Model file for the job. Use its own axes, mm. A direction names the side the tool comes from. Give positions to 0.01 mm unless a question says otherwise; leave off trailing zeros. Order: outer loops, then holes, each group sorted by start corner. A loop starts at its lowest first (then second) coordinate and runs counter-clockwise, first axis right, second up. Notation, with made-up numbers: M 34.5,78.5 L 60.5,78.5 A33 cw 60.5,113.5 Z; hole C 59,73 d4. An arc over 180 degrees is marked long. Return JSON: item names as keys, results as strings. Group by question number.
1. 3-axis set-ups, long thin cutter, end or side, ignore diameter. For faces 1 (the face through (-1, 0, 70)), 2 (the face through (-99, -4, 75)), 3 (the face through (-50, -25, 71)), 4 (the face through (98, -4, 105)): which of +Z, -Z, +X, -X, +Y, -Y reach the whole face in a straight line?
2. Wall check: probe 1 along X at (y, z) = (-3, 104); probe 2 along X at (y, z) = (1, -89); probe 3 along X at (y, z) = (4.5, 29.74). Give the ranges that are in metal, low to high. Write a range as [from, to].
3. Slice it at B-B on z = 70. List the corners of the cut face in (x, y), then the cut area to 3 significant figures.
4. Slice it at C-C on y = -21.5. List the corners of the cut face in (x, z), then the cut area to 3 significant figures.
5. Slice it at D-D on x = -102. List the corners of the cut face in (y, z).
6. Two-plate mould, pull along X, no slides. Class faces 5 (the face through (-71.45, -4, 90)), 6 (the face through (-99, -4, 105)), 7 (the face through (-125, 2, 27)), 8 (the face through (40.25, -12, 24)): released by +X, released by -X, zero draft, split by the parting line, or undercut.
7. Pin check, flat tips, straight feed: pin 1 (12 mm diameter, centred on x = -29, z = 37.5, fed in from -Y); pin 2 (12.5 mm diameter, centred on x = -4, y = -8.5, fed in from -Z); pin 3 (2 mm diameter, centred on x = 111, y = -2, fed in from +Z). Stop position of each tip, or through.
8. Slice it at A-A on x = 0. List the corners of the cut face in (y, z).
from build123d import *

# Parameters (mm, degrees)
SKETCH1_W           = 250
SKETCH1_H           = 250
BOSS_EXTRUDE1_DEPTH = 8
SKETCH2_W           = 53.55
SKETCH2_H           = 30
BOSS_EXTRUDE2_DEPTH = 7.5
SKETCH3_R           = 2.25
CUT_EXTRUDE1_DEPTH  = 178.454923854
SKETCH4_R           = 1.5
BOSS_EXTRUDE3_DEPTH = 25
FILLET1_R           = 3
CUT_EXTRUDE2_REACH  = 219.518
SKETCH5_W           = 20
SKETCH5_H           = 10
SKETCH6_R           = 1.85096309
SKETCH6_R_2         = 7.5
CUT_EXTRUDE3_DEPTH  = 20
FILLET2_R           = 10


with BuildPart() as part:
    # Sketch1 → Boss-Extrude1 (new body)
    with BuildSketch(Plane(origin=(0, 0, 0), x_dir=(1, 0, 0), z_dir=(0, 1, 0))):
        Rectangle(SKETCH1_W, SKETCH1_H)
    extrude(amount=BOSS_EXTRUDE1_DEPTH)

    # Sketch2 → Boss-Extrude2 (add)
    with BuildSketch(Plane.XZ):
        with Locations((-98.225, 90)):
            Rectangle(SKETCH2_W, SKETCH2_H)
        with Locations((98.225, 90)):
            Rectangle(SKETCH2_W, SKETCH2_H)
    extrude(amount=BOSS_EXTRUDE2_DEPTH)

    # Sketch3 → Cut-Extrude1 (cut, through all)
    with BuildSketch(Plane.XZ.offset(7.5)):
        with Locations((108.225, 90)):
            Circle(SKETCH3_R)
        with Locations((88.225, 90)):
            Circle(SKETCH3_R)
        with Locations((-108.225, 90)):
            Circle(SKETCH3_R)
        with Locations((-88.225, 90)):
            Circle(SKETCH3_R)
    extrude(amount=-CUT_EXTRUDE1_DEPTH, mode=Mode.SUBTRACT)

    # Sketch4 → Boss-Extrude3 (add)
    with BuildSketch(Plane.XZ):
        Polygon((0, 125), (-51.24999854, 125), (-51.24999854, 16.74000082), (0, 16.74000082), (51.24999854, 16.74000082), (51.24999854, 125), align=None)
        with Locations(Location((-44.24999854, 118, 0), (0, 0, 270))):
            Circle(SKETCH4_R, mode=Mode.SUBTRACT)
        with Locations(Location((44.24999854, 118, 0), (0, 0, 90))):
            Circle(SKETCH4_R, mode=Mode.SUBTRACT)
        with Locations(Location((44.24999854, 23.74000082, 0), (0, 0, 270))):
            Circle(SKETCH4_R, mode=Mode.SUBTRACT)
        with Locations(Location((-44.24999854, 23.74000082, 0), (0, 0, 90))):
            Circle(SKETCH4_R, mode=Mode.SUBTRACT)
        Polygon((0, 122), (-40.24999854, 122), (-40.24999854, 114), (-48.24999854, 114), (-48.24999854, 27.74000082), (-40.24999854, 27.74000082), (-40.24999854, 19.74000082), (0, 19.74000082), (40.24999854, 19.74000082), (40.24999854, 27.74000082), (48.24999854, 27.74000082), (48.24999854, 114), (40.24999854, 114), (40.24999854, 122), align=None, mode=Mode.SUBTRACT)
    extrude(amount=BOSS_EXTRUDE3_DEPTH)

    # Fillet1
    fillet1_edges = [part.edges().sort_by_distance(p)[0] for p in [
        (-51.24999854, 0, 70.87000041),
        (0, 0, 16.74000082),
        (-51.24999854, -12.5, 16.74000082),
        (51.24999854, 0, 70.87000041),
        (51.24999854, -12.5, 16.74000082),
    ]]
    fillet(fillet1_edges, radius=FILLET1_R)

    # Cut-Extrude2: up to this face of the body (flat: up to its plane)
    cut_extrude2_end = Plane(part.part.faces().sort_by_distance((51.24999854, -14, 72.37000041))[0])
    # Sketch5 → Cut-Extrude2 (cut, up to the picked face)
    with BuildSketch(Plane.ZY.offset(51.24999854), mode=Mode.PRIVATE) as cut_extrude2_sk1:
        with Locations((72.37000041, -8)):
            Rectangle(SKETCH5_W, SKETCH5_H)
    cut_extrude2_tool1 = split(extrude(cut_extrude2_sk1.sketch, amount=-CUT_EXTRUDE2_REACH, mode=Mode.PRIVATE), bisect_by=cut_extrude2_end, keep=Keep.BOTH, mode=Mode.PRIVATE)
    add(cut_extrude2_tool1.solids().sort_by(Axis((-51.249999, -8, 72.37), (1, 0, 0)))[0], mode=Mode.SUBTRACT)

    # Sketch6 → Cut-Extrude3 (cut)
    with BuildSketch(Plane.XZ):
        with Locations(Location((-15, -89, 0), (0, 0, 270))):
            Circle(SKETCH6_R)
        with Locations(Location((15, -89, 0), (0, 0, 270))):
            Circle(SKETCH6_R)
        with Locations(Location((15, -119, 0), (0, 0, 270))):
            Circle(SKETCH6_R)
        with Locations(Location((-15, -119, 0), (0, 0, 270))):
            Circle(SKETCH6_R)
        with Locations(Location((0, 29.74000082, 0), (0, 0, 270))):
            Circle(SKETCH6_R_2)
    extrude(amount=-CUT_EXTRUDE3_DEPTH, mode=Mode.SUBTRACT)

    # Fillet2
    fillet2_edges = [part.edges().sort_by_distance(p)[0] for p in [
        (125, 4, 125),
        (-125, 4, 125),
        (-125, 4, -125),
        (125, 4, -125),
    ]]
    fillet(fillet2_edges, radius=FILLET2_R)


solid = part.part
Result:
{
 "1": {"face 1": "-Y", "face 2": "-Z, -X, -Y", "face 3": "+Z, -Z, +X, -X, -Y", "face 4": "+Z, +X, -Y"},
 "2": {"probe 1": "x = [-125, -71.45], [-51.25, -48.25], [48.25, 51.25], [71.45, 125]", "probe 2": "x = [-125, -16.85], [-13.15, 13.15], [16.85, 125]", "probe 3": "x = [-125, -7.5], [7.5, 125]"},
 "3": {"outline": "M -125,0 L -54.25,0 A3 cw -51.25,-3 L -48.25,-3 L -48.25,0 L 48.25,0 L 48.25,-3 L 51.25,-3 A3 cw 54.25,0 L 125,0 L 125,8 L -125,8 Z; M -51.25,-25 L -48.25,-25 L -48.25,-13 L -51.25,-13 Z; M 48.25,-25 L 51.25,-25 L 51.25,-13 L 48.25,-13 Z", "area": "2,090 mm2"},
 "4": {"outline": "M -51.25,19.74 A3 ccw -48.25,16.74 L 48.25,16.74 A3 ccw 51.25,19.74 L 51.25,125 L -51.25,125 Z; hole M -48.25,27.74 L -40.25,27.74 L -40.25,19.74 L 40.25,19.74 L 40.25,27.74 L 48.25,27.74 L 48.25,114 L 40.25,114 L 40.25,122 L -40.25,122 L -40.25,114 L -48.25,114 Z; hole C -44.25,23.74 d3; hole C -44.25,118 d3; hole C 44.25,23.74 d3; hole C 44.25,118 d3", "area": "1,450 mm2"},
 "5": {"outline": "M -7.5,75 L 0,75 L 0,-125 L 8,-125 L 8,125 L 0,125 L 0,105 L -7.5,105 Z"},
 "6": {"face 5": "undercut", "face 6": "zero draft", "face 7": "released by -X", "face 8": "undercut"},
 "7": {"pin 1": "stops at y = 0", "pin 2": "stops at z = 16.64", "pin 3": "stops at z = 105"},
 "8": {"outline": "M -25,16.74 L -3,16.74 A3 cw 0,13.74 L 0,-125 L 8,-125 L 8,22.24 L 0,22.24 L 0,19.74 L -25,19.74 Z; M -25,122 L 0,122 L 0,37.24 L 8,37.24 L 8,125 L -25,125 Z"}
}
